CAD build for the part. Positions are in the model's coordinates, mm. Round coordinates to 2 decimals unless told otherwise and drop trailing zeros. Write each loop counter-clockwise with the first axis right and the second up, starting at its lowest first coordinate (ties: lowest second). Pieces come first, ordered by that corner, then holes. Notation, with made-up numbers: (79.5, 41) - (85.5, 41) arc R31 cw to (85.5, 78) - close; hole circle Ø8 at (-27.75, 44). An arc over 180 degrees is marked (long way). Answer in a Markdown table with one row per item.
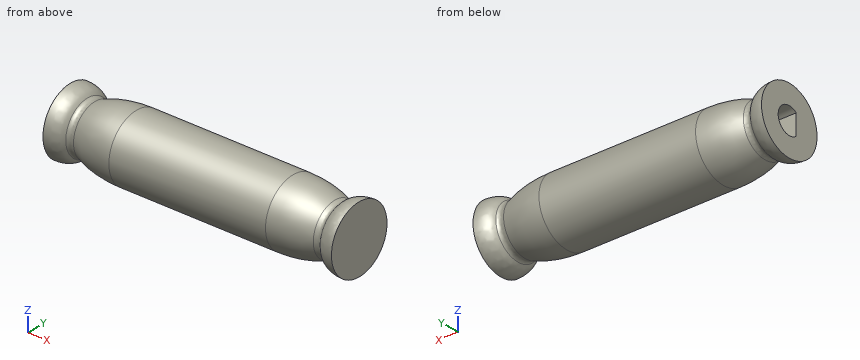
```python
from build123d import *

# Parameters (mm, degrees)
SKETCH2_R           = 4
BOSS_EXTRUDE1_DEPTH = 35
CUT_EXTRUDE1_DEPTH  = 9.8


with BuildPart() as part:
    # Sketch2 → Boss-Extrude1 (new body)
    with BuildSketch(Plane(origin=(0, 0, 0), x_dir=(0, 0, -1), z_dir=(1, 0, 0))):
        Circle(SKETCH2_R)
    extrude(amount=BOSS_EXTRUDE1_DEPTH)

    # Sketch3 → Cut-Extrude1 (cut)
    with BuildSketch(Plane.ZY):
        with BuildLine():
            Line((-1.2489996, -1), (1.2489996, -1))
            ThreePointArc((1.2489996, -1), (0, 1.6), (-1.2489996, -1))
        make_face()
    extrude(amount=-CUT_EXTRUDE1_DEPTH, mode=Mode.SUBTRACT)

    # Sketch4 → Cut-Revolve1 (revolve, cut)
    with BuildSketch(Plane.XY):
        with BuildLine():
            Line((0, 4), (8, 4))
            add(Edge.make_bspline(
                [(8, 4), (5.194687526, 4), (2.956130498, 3.107691813)],
                knots=[4.71238898, 4.71238898, 4.71238898, 5.359264748, 5.359264748, 5.359264748], degree=2, weights=[1, 0.948148367, 1]))
            add(Edge.make_bspline(
                [(2.068059433, 3.164260662), (2.318713674, 2.853611956), (2.956130498, 3.107691813)],
                knots=[0, 0, 0, 1.038649512, 1.038649512, 1.038649512], degree=2, weights=[1, 0.868154497, 1]))
            add(Edge.make_bspline(
                [(2.068059433, 3.164260662), (1.597970656, 4), (0, 4)],
                knots=[3.440188633, 3.440188633, 3.440188633, 4.71238898, 4.71238898, 4.71238898], degree=2, weights=[1, 0.804418611, 1]))
        make_face()
        with BuildLine():
            Line((27, 4), (35, 4))
            add(Edge.make_bspline(
                [(35, 4), (33.402029344, 4), (32.931940567, 3.164260662)],
                knots=[1.570796327, 1.570796327, 1.570796327, 2.842996674, 2.842996674, 2.842996674], degree=2, weights=[1, 0.804418611, 1]))
            add(Edge.make_bspline(
                [(32.043869502, 3.107691813), (32.681286326, 2.853611956), (32.931940567, 3.164260662)],
                knots=[2.102943141, 2.102943141, 2.102943141, 3.141592654, 3.141592654, 3.141592654], degree=2, weights=[1, 0.868154497, 1]))
            add(Edge.make_bspline(
                [(32.043869502, 3.107691813), (29.805312474, 4), (27, 4)],
                knots=[4.065513213, 4.065513213, 4.065513213, 4.71238898, 4.71238898, 4.71238898], degree=2, weights=[1, 0.948148367, 1]))
        make_face()
    revolve(axis=Axis((0, 0, 0), (1, 0, 0)), mode=Mode.SUBTRACT)


solid = part.part
```
Q1. Drill centre lines: line 1 (Z direction, x = 5, y = 0); line 2 (Z direction, x = 3, y = -0.5); line 3 (X direction, y = -0.75, z = -0.75). Where is each one in solid material? Low to high.
Computed:
| item | result |
|---|---|
| line 1 | z = -3.71 to -1.6, 1.6 to 3.71 |
| line 2 | z = -3.08 to -1.52, 1.52 to 3.08 |
| line 3 | x = 9.8 to 35 |
Q2. Flat gauge pins, fed straight in: pin 1 (0.8 mm diameter, centred on y = 1, z = 0, fed in from -X); pin 2 (1.5 mm diameter, centred on x = 30.5, y = 0, fed in from -Z); pin 3 (2.5 mm diameter, centred on x = 2.5, z = 0, fed in from +Y). Where does each tip first touch, or does it go through?
Computed:
| item | result |
|---|---|
| pin 1 | stops at x = 9.8 |
| pin 2 | stops at z = -3.75 |
| pin 3 | stops at y = 3.78 |
Q3. Saw through at A-A on x = 23. List the corners of the cut face in (y, z), then the cut area to 3 significant figures.
Computed:
| item | result |
|---|---|
| outline | circle Ø8 at (0, 0) |
| area | 50.3 mm2 |
